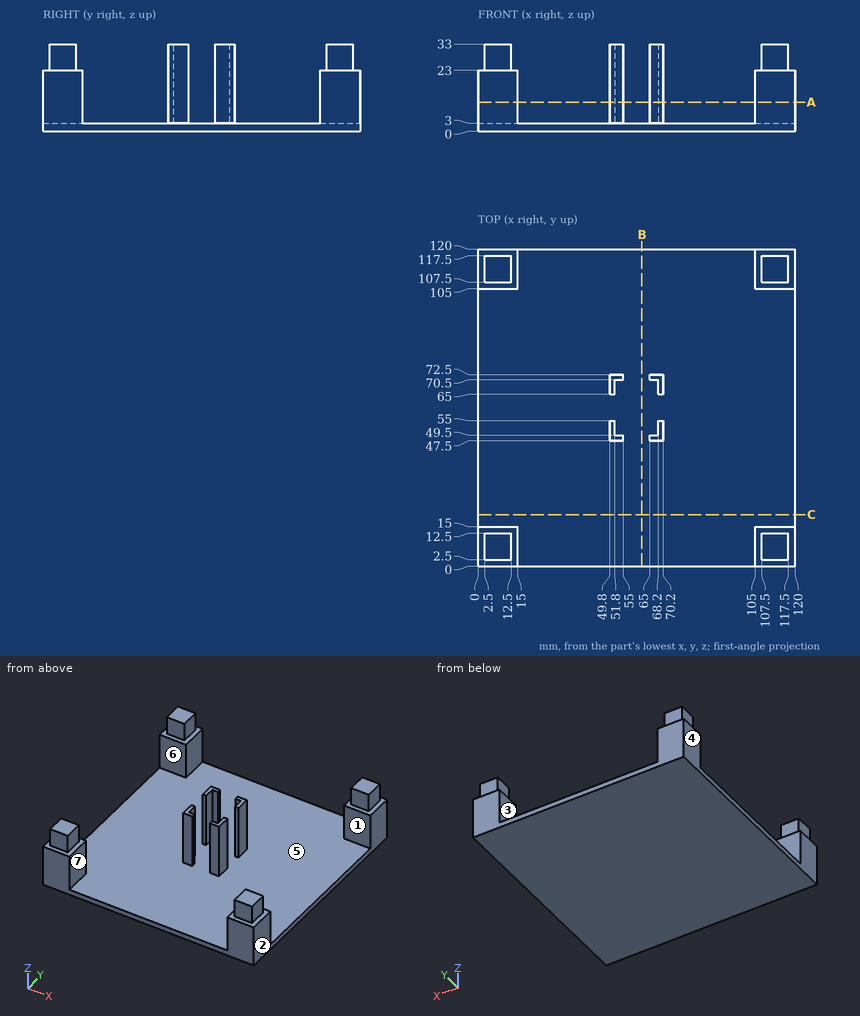
Can you work these out from the drawing? Everything is in mm from the part's minimum corner. A direction names the side the tool comes from. Coordinates: 2 decimals unless noted, no trailing zeros. Loops run counter-clockwise (first coordinate to the right, second up) from the corner with the lowest first, then second, coordinate; pieces in that order, holes last. Notation, with made-up numbers: (-33.5, -26.5) - (-1.5, -26.5) arc R30 cw to (-1.5, 2.5) - close; hole circle Ø1 at (-17, -21). An arc over 180 degrees is marked (long way). Put each result on its own line as item: value. Start each with the question number.
Item 1: Which directions (+Z, -Z, +X, -X, +Y, -Y) give clear straight access to the entire face, cutting with the end or side of a thin tool? Please do the marked faces 1, 2 and 3.
Item 2: If we mould it in two halves opening along X, with no side actions, what happens to the marked faces 4, 5, 6 and 7? For each: +X half, -X half, draft (parallel to the pull), parting line (faces both ways), or undercut.
Item 3: For pin 1 (1.6 mm diameter, centred on y = 72, z = 17.5, fed in from -X); pin 2 (1.6 mm diameter, centred on x = 51.5, z = 20.5, fed in from +Y); pin 3 (8 mm diameter, centred on y = 63.5, z = 23, fed in from +X); pin 4 (8 mm diameter, centred on y = 40, z = 24, fed in from +X), each with a flat end and sliding along its axis, tell me the tip position at first contact or that it passes through.
Item 4: Suppose I cut it at A-A (z = 11). State how many separate pieces and enclosed holes the cut face has, and give its area (3 significant figures).
Item 5: Suppose I cut it at B-B (x = 62). Please give me the cut outline in (y, z), and give its area (3 significant figures).
Item 6: If I drill on line 1 along Y through (x, z) = (53.5, 13.5); line 2 along Y through (x, z) = (109, 4.5); line 3 along Z through (x, y) = (35.5, 42), over which ranges is the centre line in solid material (lowest first)?
Here are the results:
1. face 1: +Z, +X, -X
1. face 2: +Z, -Z, +X, +Y, -Y
1. face 3: +Z, +Y, -Y
2. face 4: -X half
2. face 5: undercut
2. face 6: draft
2. face 7: undercut
3. pin 1: x = 49.8
3. pin 2: y = 72.5
3. pin 3: x = 70.2
3. pin 4: through
4. separate pieces: 8
4. enclosed holes: 0
4. area: 986 mm²
5. outline: (0, 0) - (120, 0) - (120, 3) - (0, 3) - close
5. area: 360 mm²
6. line 1: 47.5 to 49.5, 70.5 to 72.5
6. line 2: 0 to 15, 105 to 120
6. line 3: 0 to 3
